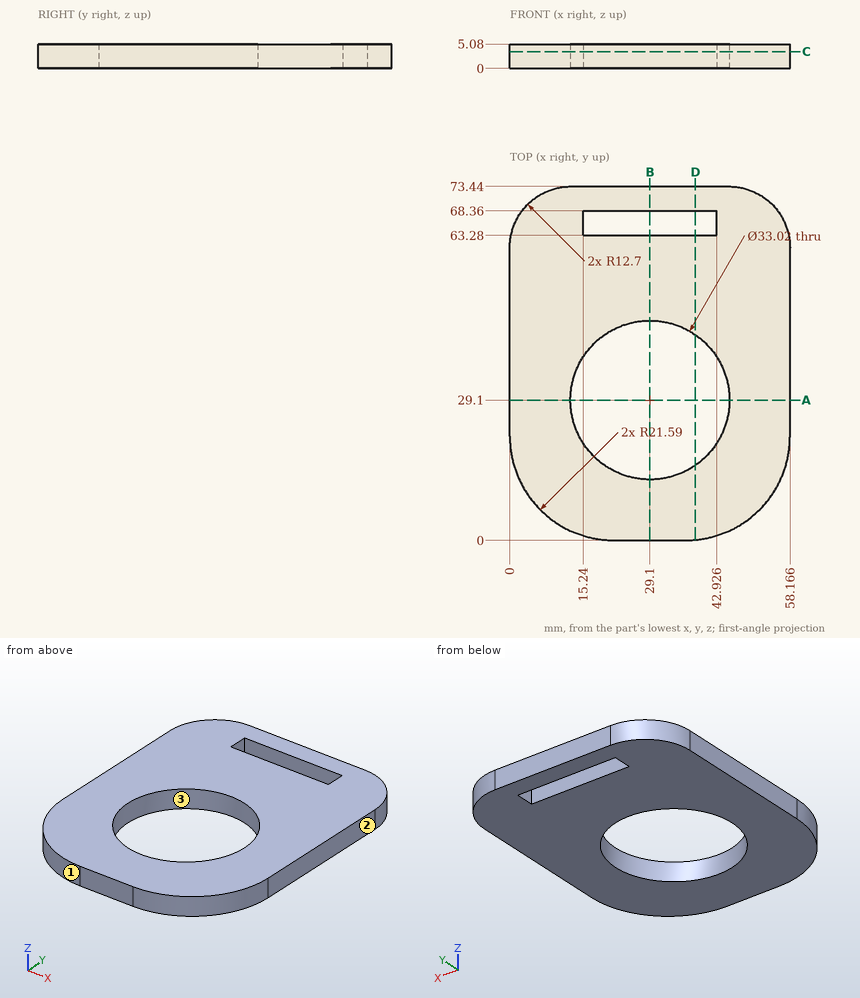
Geometry: see drawing. Coordinates: mm, zero at the bounding-box minimum. Give positions to 0.01 mm unless a question says otherwise; leave off trailing zeros. Write each loop counter-clockwise with the first axis right and the second up, starting at its lowest first coordinate (ties: lowest second). Pieces come first, ordered by that corner, then holes. Notation, with made-up numbers: M 75.5,87 L 96.5,87 A21 ccw 96.5,98 Z; hole C 30,45.25 d4. An arc over 180 degrees is marked long. Return JSON: item names as keys, results as strings. Group by question number.
1) Cut plane D-D, the plane x = 38.5. Output: boundary loops of the cut face in (y, z).
2) Ray query, L1, parallel to Y at x = 29.1, z = 4.05; L2, parallel to Y at x = 24.5, z = 1.45; L3, parallel to X at y = 43.5, z = 4.5. Return the intervals inside material, ascending.
3) First-contact query: pin 1 Ø2 at (y, z) = (41, 2.5) entering from -X; pin 2 Ø1 at (x, z) = (7, 2.5) entering from +Y; pin 3 Ø3 at (x, z) = (14, 2) entering from -Y; pin 4 Ø2.5 at (y, z) = (65, 1.5) entering from -X. Flat tips, straight axial feed; report the tip coordinate or a pass-through.
4) Cut plane A-A, the plane y = 29.1. Output: boundary loops of the cut face in (x, z).
5) Draft query along X for the marked faces 1, 2 and 3. Return one class per face: released by +X, released by -X, zero draft, split by the parting line, or undercut.
6) Cut plane B-B, the plane x = 29.1. Output: boundary loops of the cut face in (y, z), then the cut area to 3 significant figures.
7) Cut plane C-C, the plane z = 3.5. Output: boundary loops of the cut face in (x, y), then the cut area to 3 significant figures.
Data:
{
 "1": {"outline": "M 0.09,0 L 15.53,0 L 15.53,5.08 L 0.09,5.08 Z; M 42.67,0 L 63.28,0 L 63.28,5.08 L 42.67,5.08 Z; M 68.36,0 L 73.44,0 L 73.44,5.08 L 68.36,5.08 Z"},
 "2": {"L1": "y = 0 to 12.59, 45.61 to 63.28, 68.36 to 73.44", "L2": "y = 0 to 13.24, 44.96 to 63.28, 68.36 to 73.44", "L3": "x = 0 to 21.02, 37.18 to 58.17"},
 "3": {"pin 1": "stops at x = 0", "pin 2": "stops at y = 72.33", "pin 3": "stops at y = 0.88", "pin 4": "stops at x = 0.36"},
 "4": {"outline": "M 0,0 L 12.59,0 L 12.59,5.08 L 0,5.08 Z; M 45.61,0 L 58.17,0 L 58.17,5.08 L 45.61,5.08 Z"},
 "5": {"face 1": "released by -X", "face 2": "released by +X", "face 3": "undercut"},
 "6": {"outline": "M 0,0 L 12.59,0 L 12.59,5.08 L 0,5.08 Z; M 45.61,0 L 63.28,0 L 63.28,5.08 L 45.61,5.08 Z; M 68.36,0 L 73.44,0 L 73.44,5.08 L 68.36,5.08 Z", "area": "180 mm²"},
 "7": {"outline": "M 0,21.59 A21.59 ccw 21.59,0 L 36.58,0 A21.59 ccw 58.17,21.59 L 58.17,60.74 A12.7 ccw 45.47,73.44 L 12.7,73.44 A12.7 ccw 0,60.74 Z; hole C 29.1,29.1 d33.02; hole M 15.24,63.28 L 42.93,63.28 L 42.93,68.36 L 15.24,68.36 Z", "area": "3,010 mm²"}
}
